The model under review builds one solid part; all positions refer to its coordinate system, in mm. A direction names the side the tool comes from. Round coordinates to 2 decimals unless told otherwise and drop trailing zeros. Order: outer loops, then holes, each group sorted by start corner. A loop starts at its lowest first (then second) coordinate and runs counter-clockwise, first axis right, second up.
from build123d import *

# Parameters (mm, degrees)
BOSS_EXTRUDE1_DEPTH     = 10
CUT_EXTRUDE1_DEPTH      = 47.99468055
SKETCH8_W               = 5.5
SKETCH8_H               = 5
CUT_EXTRUDE7_DEPTH      = 47.99468055
CUT_EXTRUDE8_DEPTH      = 52.994106262
CUT_EXTRUDE8_DEPTH_BACK = 52.994106262
SKETCH9_W               = 4
SKETCH9_H               = 5.5
FILLET4_R               = 1.5
CUT_EXTRUDE9_DEPTH      = 5.5
CHAMFER1_SIZE           = 4
SKETCH11_W              = 11
SKETCH11_H              = 16.199337742
SKETCH11_W_2            = 4
SKETCH11_H_2            = 6
CUT_EXTRUDE10_DEPTH     = 47.99468055
FILLET5_R               = 12


with BuildPart() as part:
    # Sketch1 → Boss-Extrude1 (new body)
    with BuildSketch(Plane.XY):
        with BuildLine():
            Line((-26.5, -8.099668871), (-26.5, -15.099668871))
            ThreePointArc((-26.5, -15.099668871), (-21.566756826, -21.566756826), (-15.099668871, -26.5))
            Line((-15.099668871, -26.5), (0, -26.5))
            Line((0, -26.5), (0, -21.5))
            Line((0, -21.5), (-13.711309201, -21.5))
            ThreePointArc((-13.711309201, -21.5), (-18.03122292, -18.03122292), (-21.5, -13.711309201))
            Line((-21.5, -13.711309201), (-21.5, 13.711309201))
            ThreePointArc((-21.5, 13.711309201), (-18.03122292, 18.03122292), (-13.711309201, 21.5))
            Line((-13.711309201, 21.5), (0, 21.5))
            Line((0, 21.5), (0, 26.5))
            Line((0, 26.5), (-15.099668871, 26.5))
            ThreePointArc((-15.099668871, 26.5), (-21.566756826, 21.566756826), (-26.5, 15.099668871))
            Line((-26.5, 15.099668871), (-26.5, 8.099668871))
            Line((-26.5, 8.099668871), (-37.5, 8.099668871))
            Line((-37.5, 8.099668871), (-37.5, -8.099668871))
            Line((-37.5, -8.099668871), (-26.5, -8.099668871))
        make_face()
    extrude(amount=BOSS_EXTRUDE1_DEPTH)

    # Sketch2 → Cut-Extrude1 (cut, through all)
    with BuildSketch(Plane.XY.offset(10)):
        with BuildLine():
            Line((-31, 2.907722565), (-31, -2.907722565))
            ThreePointArc((-31, -2.907722565), (-33, -4.907722565), (-35, -2.907722565))
            Line((-35, -2.907722565), (-35, 2.907722565))
            ThreePointArc((-35, 2.907722565), (-33, 4.907722565), (-31, 2.907722565))
        make_face()
    extrude(amount=-CUT_EXTRUDE1_DEPTH, mode=Mode.SUBTRACT)

    # Sketch8 → Cut-Extrude7 (cut, through all)
    with BuildSketch(Plane(origin=(0, 0, 0), x_dir=(0, 0, -1), z_dir=(1, 0, 0))):
        with Locations((-5, 26.5)):
            Rectangle(SKETCH8_W, SKETCH8_H)
        with Locations((-5, -26.5)):
            Rectangle(SKETCH8_W, SKETCH8_H)
    extrude(amount=-CUT_EXTRUDE7_DEPTH, mode=Mode.SUBTRACT)

    # Sketch9 → Cut-Extrude8 (cut, two sides: drawn at the far end of the back side and taken through both)
    with BuildSketch(Plane.XZ.offset(8.099668871).offset(-CUT_EXTRUDE8_DEPTH_BACK)):
        with Locations((-26.5, 5)):
            Rectangle(SKETCH9_W, SKETCH9_H)
    extrude(amount=CUT_EXTRUDE8_DEPTH + CUT_EXTRUDE8_DEPTH_BACK, mode=Mode.SUBTRACT)

    # Fillet4
    fillet4_edges = [part.edges().sort_by_distance(p)[0] for p in [
        (-28.5, 0, 2.25),
        (-28.5, 0, 7.75),
    ]]
    fillet(fillet4_edges, radius=FILLET4_R)

    # Sketch10 → Cut-Extrude9 (cut)
    with BuildSketch(Plane.XY.offset(2.25)):
        with BuildLine():
            Line((-16.314836512, 24), (-18.821530225, 24))
            ThreePointArc((-18.821530225, 24), (-21.856301603, 21.273271498), (-24.5, 18.165902125))
            Line((-24.5, 18.165902125), (-24.5, 15.08975312))
            ThreePointArc((-24.5, 15.08975312), (-20.789536476, 19.895899393), (-16.314836512, 24))
        make_face()
        with BuildLine():
            Line((-24.5, -15.08975312), (-24.5, -18.165902125))
            ThreePointArc((-24.5, -18.165902125), (-21.856301603, -21.273271498), (-18.821530225, -24))
            Line((-18.821530225, -24), (-16.314836512, -24))
            ThreePointArc((-16.314836512, -24), (-20.789536476, -19.895899393), (-24.5, -15.08975312))
        make_face()
    extrude(amount=CUT_EXTRUDE9_DEPTH, mode=Mode.SUBTRACT)

    # Chamfer1
    chamfer1_edges = [part.edges().sort_by_distance(p)[0] for p in [
        (0, -26.5, 8.875),
        (0, 26.5, 8.875),
    ]]
    chamfer(chamfer1_edges, length=CHAMFER1_SIZE)

    # Sketch11 → Cut-Extrude10 (cut, through all)
    with BuildSketch(Plane(origin=(0, 0, 0), x_dir=(-1, 0, 0), z_dir=(0, 0, -1))):
        with Locations((32, 0)):
            Rectangle(SKETCH11_W, SKETCH11_H)
        with Locations((21.5, 0)):
            Rectangle(SKETCH11_W_2, SKETCH11_H_2)
    extrude(amount=-CUT_EXTRUDE10_DEPTH, mode=Mode.SUBTRACT)

    # Fillet5
    fillet5_edges = [part.edges().sort_by_distance(p)[0] for p in [
        (-24.5, 15.08975312, 5),
        (-16.314836512, 24, 5),
        (-16.314836512, -24, 5),
        (-24.5, -15.08975312, 5),
    ]]
    fillet(fillet5_edges, radius=FILLET5_R)


solid = part.part
(1) We need section D-D (x = -8.75). Give the boundary of the cut face in (y, z).
(2) To check wall thickness, follow L1, parallel to Y at x = -9, z = 4.5; L2, parallel to Z at x = -20.25, y = -20.5; L3, parallel to Y at x = -4.5, z = 8.75. State the ranges of each line that lie inside material, in increasing order.
(3) Tool access review of faces 1 (the cylindrical face through (-16.56, -22.99, 5.04)), 2 (the flat face through (-7, -24, 5)), 3 (the flat face through (-7, -21.5, 5)), 4 (the flat face through (-25, 0, 7.75)): name each direction out of +Z, -Z, +X, -X, +Y, -Y from which nothing blocks a thin tool from reaching the whole face with its end or side.
(4) The part is to be moulded in two halves that separate along Y. For faces 5 (the cylindrical face through (-21.486, 21.647, 1.109)), 6 (the flat face through (-21.5, -8, 5)), 7 (the flat face through (0, 22, 5)), say which applies: pulls with the +Y half, pulls with the -Y half, needs draft (parallel to the pull), parting line crosses it, or undercut.
(5) We need section B-B (z = 3.5). Give the boundary of the cut face in (x, y), and give its area (3 significant figures).
(6) We need section C-C (y = 2). Give the boundary of the cut face in (x, z), and give its area (3 significant figures).
(7) We need section A-A (x = -23). Give the boundary of the cut face in (y, z).
(8) Clearance check with flat-ended pins moving along their axes: P1, Ø1, axis at x = -23.5, z = 1.5, coming from the +Y side; P2, Ø3, axis at y = 8.5, z = 4.5, coming from the +X side; P3, Ø1.6, axis at x = -23, z = 5.5, coming from the -Y side. State where each tip first meets the part, or that it passes through.
Verdict:
1. outline: (-26.5, 0) - (-21.5, 0) - (-21.5, 10) - (-26.5, 10) - (-26.5, 7.75) - (-24, 7.75) - (-24, 2.25) - (-26.5, 2.25) - close; (21.5, 0) - (26.5, 0) - (26.5, 2.25) - (24, 2.25) - (24, 7.75) - (26.5, 7.75) - (26.5, 10) - (21.5, 10) - close
2. L1: y = -24 to -21.5, 21.5 to 24
2. L2: z = 0 to 2.25, 7.75 to 10
2. L3: y = -26.5 to -21.5, 21.5 to 26.5
3. face 1: -X, -Y
3. face 2: +X, -X, -Y
3. face 3: +Z, -Z, +X
3. face 4: -X
4. face 5: pulls with the +Y half
4. face 6: undercut
4. face 7: needs draft
5. outline: (-24.5, -11.16) arc R12 ccw to (-21.62, -18.96) arc R35.53 ccw to (-20.48, -20.23) arc R12 ccw to (-11.75, -24) - (-1.5, -24) - (0, -22.5) - (0, -21.5) - (-13.71, -21.5) arc R25.5 cw to (-21.5, -13.71) - (-21.5, -3) - (-23.5, -3) - (-23.5, 3) - (-21.5, 3) - (-21.5, 13.71) arc R25.5 cw to (-13.71, 21.5) - (0, 21.5) - (0, 22.5) - (-1.5, 24) - (-11.75, 24) arc R12 ccw to (-20.48, 20.23) arc R35.53 ccw to (-21.62, 18.96) arc R12 ccw to (-24.5, 11.16) - close
5. area: 215 mm2
6. outline: (-26.5, 0) - (-23.5, 0) - (-23.5, 10) - (-26.5, 10) - (-26.5, 7.75) - (-24.5, 7.75) - (-24.5, 2.25) - (-26.5, 2.25) - close
6. area: 19.0 mm2
7. outline: (-20.03, 0) - (-3, 0) - (-3, 10) - (-20.03, 10) - (-20.03, 7.75) - (-16.97, 7.75) - (-16.97, 2.25) - (-20.03, 2.25) - close; (3, 0) - (20.03, 0) - (20.03, 2.25) - (16.97, 2.25) - (16.97, 7.75) - (20.03, 7.75) - (20.03, 10) - (3, 10) - close
8. P1: stops at y = 20.03
8. P2: stops at x = -21.5
8. P3: stops at y = -18.22
